Source: three-view drawing plus pictorial views. Frame: mm from the lowest corner of the part. A direction names the side the tool comes from. Round coordinates to 2 decimals unless told otherwise and drop trailing zeros. Loops run counter-clockwise (first coordinate to the right, second up) from the corner with the lowest first, then second, coordinate; pieces in that order, holes last. Notation, with made-up numbers: (13, 21.5) -> (53, 21.5) arc R18 ccw to (53, 32.5) -> close; hole circle Ø3 at (52, 44.25). An arc over 180 degrees is marked (long way). Put each result on its own line as item: value. Start each with the question number.
1. Draft query along X for the marked faces 4, 5 and 6. Return one class per face: pulls with the +X half, pulls with the -X half, needs draft (parallel to the pull), parting line crosses it, or undercut.
2. Cut plane A-A (x = 3). Return the cut outline in (y, z), then the cut area to 3 significant figures.
3. Set-up query: the marked faces 1, 2 and 3. Return all of +Z, -Z, +X, -X, +Y, -Y with unobstructed straight access to the full face (end or side cutting, diameter ignored); none if empty.
4. Cut plane B-B (z = 3). Return the cut outline in (x, y), then the cut area to 3 significant figures.
5. Contact query for flat-ended pins moving along their axis: pin 1 (1.9 mm diameter, centred on x = 3, z = 3, fed in from +Y); pin 2 (3 mm diameter, centred on x = 1, z = 1, fed in from +Y). Output: stop coordinate, or through.
6. Cut plane D-D (y = 6.25). Return the cut outline in (x, z).
7. Cut plane C-C (y = 4.5). Return the cut outline in (x, z).
8. Material intervals for L1, parallel to Z at x = 3, y = 6.15; L2, parallel to Y at x = 5.4, z = 2.55; L3, parallel to X at y = 1, z = 3.05, sorted ascending.
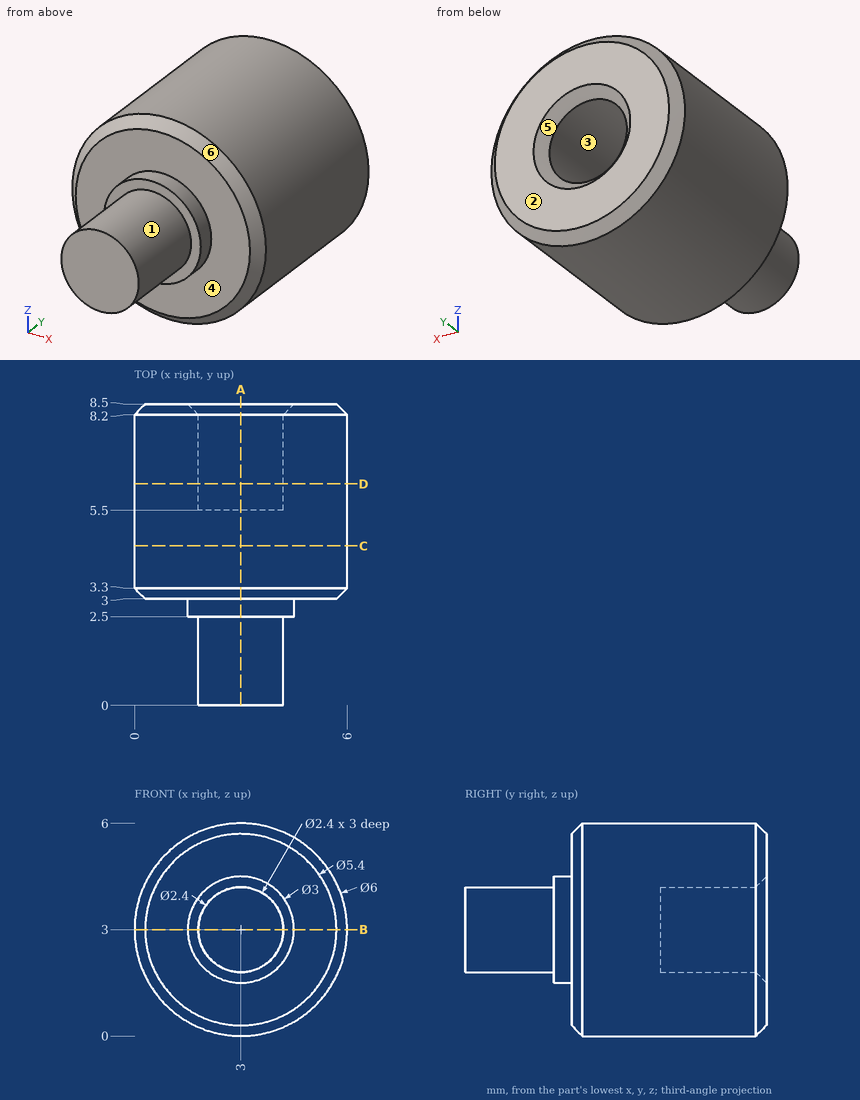
Solution:
1. face 4: needs draft
1. face 5: undercut
1. face 6: parting line crosses it
2. outline: (0, 1.8) -> (2.5, 1.8) -> (2.5, 1.5) -> (3, 1.5) -> (3, 0.3) -> (3.3, 0) -> (8.2, 0) -> (8.5, 0.3) -> (8.5, 1.5) -> (8.2, 1.8) -> (5.5, 1.8) -> (5.5, 4.2) -> (8.2, 4.2) -> (8.5, 4.5) -> (8.5, 5.7) -> (8.2, 6) -> (3.3, 6) -> (3, 5.7) -> (3, 4.5) -> (2.5, 4.5) -> (2.5, 4.2) -> (0, 4.2) -> close
2. area: 33.0 mm^2
3. face 1: -Y
3. face 2: +Z, -Z, +X, -X, +Y
3. face 3: +Y
4. outline: (0, 3.3) -> (0.3, 3) -> (1.5, 3) -> (1.5, 2.5) -> (1.8, 2.5) -> (1.8, 0) -> (4.2, 0) -> (4.2, 2.5) -> (4.5, 2.5) -> (4.5, 3) -> (5.7, 3) -> (6, 3.3) -> (6, 8.2) -> (5.7, 8.5) -> (4.5, 8.5) -> (4.2, 8.2) -> (4.2, 5.5) -> (1.8, 5.5) -> (1.8, 8.2) -> (1.5, 8.5) -> (0.3, 8.5) -> (0, 8.2) -> close
4. area: 33.0 mm^2
5. pin 1: stops at y = 5.5
5. pin 2: stops at y = 8.5
6. outline: circle Ø6 at (3, 3); hole circle Ø2.4 at (3, 3)
7. outline: circle Ø6 at (3, 3)
8. L1: z = 0 to 1.8, 4.2 to 6
8. L2: y = 3 to 8.5
8. L3: x = 1.8 to 4.2
